The model under review builds one solid part; all positions refer to its coordinate system, in mm. A direction names the side the tool comes from. Round coordinates to 2 decimals unless told otherwise and drop trailing zeros. Write each loop counter-clockwise with the first axis right and the second up, starting at its lowest first coordinate (ties: lowest second). Pieces come first, ordered by that corner, then holes. Notation, with made-up numbers: (62.25, 64) -> (76.25, 64) arc R35 ccw to (76.25, 98) -> close; hole circle Ø9 at (70.25, -4). An arc over 180 degrees is marked (long way). Return JSON: item names as keys, results as strings. Group by question number.
1. Take a section at D-D, the plane y = 3.5. Write out the cut boundary in (x, z).
2. Take a section at C-C, the plane x = 4.75. Write out the cut boundary in (y, z).
3. Tool access review of faces 1 (the cylindrical face through (-1.689, 12.457, -0.651)), 2 (the flat face through (0, 15, 0)): name each direction out of +Z, -Z, +X, -X, +Y, -Y from which nothing blocks a thin tool from reaching the whole face with its end or side.
4. Mouldability with a two-part tool opening along Y and no side actions: class faces 3 (the flat face through (13.5, 7.4, 6)), 4 (the flat face through (0, 0, 0)), 5 (the flat face through (12, 9, 0)) as pulls with the +Y half, pulls with the -Y half, needs draft (parallel to the pull), parting line crosses it, or undercut.
5. Take a section at A-A, the plane y = 7.5. Write out the cut boundary in (x, z).
6. Clearance check with a flat-ended pin moving along its axis: P1, Ø3, axis at y = 7.5, z = 0, coming from the -X side. State where the tip first meets the part, or that it passes through.
7. Take a section at B-B, the plane z = 0. Write out the cut boundary in (x, y), then the cut area to 3 significant figures.
8. For line 1 along Y through (x, z) = (14, 0); line 2 along Y through (x, z) = (7.75, 0.25); line 3 along Z through (x, y) = (5.5, 11.5), list the stretches that pass through material, from the lowest coordinate up. Write a range as from..to.
from build123d import *

# Parameters (mm, degrees)
SKETCH1_W           = 30
SKETCH1_H           = 15
BOSS_EXTRUDE1_DEPTH = 15
CHAMFER1_SIZE       = 3
SKETCH2_R           = 5
CUT_EXTRUDE1_DEPTH  = 27
SKETCH3_R           = 1.15
CUT_EXTRUDE2_DEPTH  = 7


with BuildPart() as part:
    # Sketch1 → Boss-Extrude1 (new body)
    with BuildSketch(Plane(origin=(0, 0, 0), x_dir=(1, 0, 0), z_dir=(0, 1, 0))):
        Rectangle(SKETCH1_W, SKETCH1_H)
    extrude(amount=BOSS_EXTRUDE1_DEPTH)

    # Chamfer1
    chamfer1_edges = [part.edges().sort_by_distance(p)[0] for p in [
        (15, 7.5, 7.5),
        (15, 7.5, -7.5),
    ]]
    chamfer(chamfer1_edges, length=CHAMFER1_SIZE)

    # Sketch2 → Cut-Extrude1 (cut)
    with BuildSketch(Plane.ZY.offset(15)):
        with Locations((0, 7.5)):
            Circle(SKETCH2_R)
    extrude(amount=-CUT_EXTRUDE1_DEPTH, mode=Mode.SUBTRACT)

    # Sketch3 → Cut-Extrude2 (cut)
    with BuildSketch(Plane.ZY.offset(-12)):
        with Locations((0, 7.5)):
            Circle(SKETCH3_R)
    extrude(amount=-CUT_EXTRUDE2_DEPTH, mode=Mode.SUBTRACT)


solid = part.part
Output:
{
 "1": {"outline": "(-15, -7.5) -> (12, -7.5) -> (15, -4.5) -> (15, 4.5) -> (12, 7.5) -> (-15, 7.5) -> (-15, 3) -> (12, 3) -> (12, -3) -> (-15, -3) -> close"},
 "2": {"outline": "(0, -7.5) -> (15, -7.5) -> (15, 7.5) -> (0, 7.5) -> close; hole circle Ø10 at (7.5, 0)"},
 "3": {"face 1": "-X", "face 2": "+Z, -Z, +X, -X, +Y"},
 "4": {"face 3": "needs draft", "face 4": "pulls with the -Y half", "face 5": "undercut"},
 "5": {"outline": "(-15, -7.5) -> (12, -7.5) -> (15, -4.5) -> (15, -1.15) -> (12, -1.15) -> (12, -5) -> (-15, -5) -> close; (-15, 5) -> (12, 5) -> (12, 1.15) -> (15, 1.15) -> (15, 4.5) -> (12, 7.5) -> (-15, 7.5) -> close"},
 "6": {"P1": "stops at x = 12"},
 "7": {"outline": "(-15, 0) -> (15, 0) -> (15, 6.35) -> (12, 6.35) -> (12, 2.5) -> (-15, 2.5) -> close; (-15, 12.5) -> (12, 12.5) -> (12, 8.65) -> (15, 8.65) -> (15, 15) -> (-15, 15) -> close", "area": "173 mm^2"},
 "8": {"line 1": "y = 0..6.35, 8.65..15", "line 2": "y = 0..2.51, 12.49..15", "line 3": "z = -7.5..-3, 3..7.5"}
}
